Source: CAD feature listing. Evaluate the final solid. Frame: model axes, mm. A direction names the side the tool comes from. Give positions to 0.01 mm unless a question says otherwise; leave off trailing zeros. Loops run counter-clockwise (first coordinate to the right, second up) from the corner with the lowest first, then second, coordinate; pieces in that order, holes last. Notation, with made-up numbers: M -11,-40 L 5,-40 A27 ccw 5,-8 Z; hole C 53,82 d6. An arc over 180 degrees is marked long. Put each result on its own line as item: value.
from build123d import *

# Parameters (mm, degrees)
SKETCH1_W           = 28.2
SKETCH1_H           = 28.2
SKETCH1_R           = 11.1
SKETCH1_R_2         = 1.5
SKETCH1_R_3         = 5.2
BOSS_EXTRUDE1_DEPTH = 25
SKETCH1_4_R         = 5.2
CUT_EXTRUDE1_DEPTH  = 25
SKETCH1_5_R         = 1.5
CUT_EXTRUDE2_DEPTH  = 8
SKETCH1_6_R         = 11.1
SKETCH1_6_R_2       = 1.5
SKETCH1_6_R_3       = 5.2
CUT_EXTRUDE3_DEPTH  = 3.5
SKETCH2_R           = 1.5
CUT_EXTRUDE4_DEPTH  = 5


with BuildPart() as part:
    # Sketch1 → Boss-Extrude1 (new body)
    # profile 1 of 7: a face of its own
    with BuildSketch(Plane(origin=(0, 0, 0), x_dir=(1, 0, 0), z_dir=(0, 1, 0))):
        Rectangle(SKETCH1_W, SKETCH1_H)
        Circle(SKETCH1_R, mode=Mode.SUBTRACT)
    # profile 2 of 7: a face of its own
    with BuildSketch(Plane(origin=(0, 0, 0), x_dir=(1, 0, 0), z_dir=(0, 1, 0))):
        Circle(SKETCH1_R)
        with Locations((8, 0)):
            Circle(SKETCH1_R_2, mode=Mode.SUBTRACT)
        with Locations((0, -8)):
            Circle(SKETCH1_R_2, mode=Mode.SUBTRACT)
        with Locations((-8, 0)):
            Circle(SKETCH1_R_2, mode=Mode.SUBTRACT)
        with Locations((0, 8)):
            Circle(SKETCH1_R_2, mode=Mode.SUBTRACT)
        Circle(SKETCH1_R_3, mode=Mode.SUBTRACT)
    # profile 3 of 7: a face of its own
    with BuildSketch(Plane(origin=(0, 0, 0), x_dir=(1, 0, 0), z_dir=(0, 1, 0))):
        with Locations((0, 8)):
            Circle(SKETCH1_R_2)
    # profile 4 of 7: a face of its own
    with BuildSketch(Plane(origin=(0, 0, 0), x_dir=(1, 0, 0), z_dir=(0, 1, 0))):
        with Locations((8, 0)):
            Circle(SKETCH1_R_2)
    # profile 5 of 7: a face of its own
    with BuildSketch(Plane(origin=(0, 0, 0), x_dir=(1, 0, 0), z_dir=(0, 1, 0))):
        with Locations((0, -8)):
            Circle(SKETCH1_R_2)
    # profile 6 of 7: a face of its own
    with BuildSketch(Plane(origin=(0, 0, 0), x_dir=(1, 0, 0), z_dir=(0, 1, 0))):
        with Locations((-8, 0)):
            Circle(SKETCH1_R_2)
    # profile 7 of 7: a face of its own
    with BuildSketch(Plane(origin=(0, 0, 0), x_dir=(1, 0, 0), z_dir=(0, 1, 0))):
        Circle(SKETCH1_R_3)
    extrude(amount=BOSS_EXTRUDE1_DEPTH)

    # Sketch1_4 → Cut-Extrude1 (cut)
    with BuildSketch(Plane(origin=(0, 0, 0), x_dir=(1, 0, 0), z_dir=(0, 1, 0))):
        with Locations(Location((0, 0, 0), (0, 0, 270))):
            Circle(SKETCH1_4_R)
    extrude(amount=CUT_EXTRUDE1_DEPTH, mode=Mode.SUBTRACT)

    # Sketch1_5 → Cut-Extrude2 (cut)
    with BuildSketch(Plane(origin=(0, 0, 0), x_dir=(1, 0, 0), z_dir=(0, 1, 0))):
        with Locations(Location((-8, 0, 0), (0, 0, 270))):
            Circle(SKETCH1_5_R)
        with Locations(Location((0, -8, 0), (0, 0, 270))):
            Circle(SKETCH1_5_R)
        with Locations(Location((8, 0, 0), (0, 0, 270))):
            Circle(SKETCH1_5_R)
        with Locations(Location((0, 8, 0), (0, 0, 270))):
            Circle(SKETCH1_5_R)
    extrude(amount=CUT_EXTRUDE2_DEPTH, mode=Mode.SUBTRACT)

    # Sketch1_6 → Cut-Extrude3 (cut)
    with BuildSketch(Plane(origin=(0, 0, 0), x_dir=(1, 0, 0), z_dir=(0, 1, 0))):
        with Locations(Location((0, 0, 0), (0, 0, 270))):
            Circle(SKETCH1_6_R)
        with Locations(Location((8, 0, 0), (0, 0, 270))):
            Circle(SKETCH1_6_R_2, mode=Mode.SUBTRACT)
        with Locations(Location((0, -8, 0), (0, 0, 270))):
            Circle(SKETCH1_6_R_2, mode=Mode.SUBTRACT)
        with Locations(Location((-8, 0, 0), (0, 0, 270))):
            Circle(SKETCH1_6_R_2, mode=Mode.SUBTRACT)
        with Locations(Location((0, 8, 0), (0, 0, 270))):
            Circle(SKETCH1_6_R_2, mode=Mode.SUBTRACT)
        with Locations(Location((0, 0, 0), (0, 0, 270))):
            Circle(SKETCH1_6_R_3, mode=Mode.SUBTRACT)
    extrude(amount=CUT_EXTRUDE3_DEPTH, mode=Mode.SUBTRACT)

    # Sketch2 → Cut-Extrude4 (cut)
    with BuildSketch(Plane.ZY.offset(14.1)):
        with Locations((-7.5, 20.5)):
            Circle(SKETCH2_R)
        with Locations((7.5, 20.5)):
            Circle(SKETCH2_R)
        with Locations((7.5, 4.5)):
            Circle(SKETCH2_R)
        with Locations((-7.5, 4.5)):
            Circle(SKETCH2_R)
    extrude(amount=-CUT_EXTRUDE4_DEPTH, mode=Mode.SUBTRACT)


solid = part.part
1. Draft query along X for faces 1 (the cylindrical face through (-11.64, 21.51, -8.61)), 2 (the cylindrical face through (6.536, 5.719, -0.325)), 3 (the flat face through (-9.1, 21, 7)). Return one class per face: pulls with the +X half, pulls with the -X half, needs draft (parallel to the pull), parting line crosses it, or undercut.
Found:
face 1: needs draft
face 2: undercut
face 3: pulls with the -X half
2. Section query C-C (z = 0). Output: boundary loops of the cut face in (x, y).
Found:
outline: M -14.1,0 L -11.1,0 L -11.1,3.5 L -9.5,3.5 L -9.5,8 L -6.5,8 L -6.5,3.5 L -5.2,3.5 L -5.2,25 L -14.1,25 Z; M 5.2,3.5 L 6.5,3.5 L 6.5,8 L 9.5,8 L 9.5,3.5 L 11.1,3.5 L 11.1,0 L 14.1,0 L 14.1,25 L 5.2,25 Z
3. Material intervals for line 1 (X direction, y = 4.85, z = 0); line 2 (Y direction, x = -11.6, z = -7.5); line 3 (X direction, y = 0.7, z = 0), sorted ascending. Write a range as from..to.
Found:
line 1: -14.1..-9.5, -6.5..-5.2, 5.2..6.5, 9.5..14.1
line 2: 0..3, 6..19, 22..25
line 3: -14.1..-11.1, 11.1..14.1
4. Section query D-D (x = 8). Output: boundary loops of the cut face in (y, z).
Found:
outline: M 0,-14.1 L 25,-14.1 L 25,14.1 L 0,14.1 L 0,7.69 L 3.5,7.69 L 3.5,1.5 L 8,1.5 L 8,-1.5 L 3.5,-1.5 L 3.5,-7.69 L 0,-7.69 Z
5. Contact query for flat-ended pins moving along their axis: P1, Ø5, axis at x = 0, z = 8, coming from the -Y side; P2, Ø1.5, axis at y = 20.5, z = -7.5, coming from the -X side; P3, Ø6, axis at x = 0, z = 0, coming from the -Y side; P4, Ø1.5, axis at x = -7.5, z = 0, coming from the -Y side. Output: stop coordinate, or through.
Found:
P1: y = 3.5
P2: x = -9.1
P3: through
P4: y = 8
6. Section query A-A (y = 14.5). Output: boundary loops of the cut face in (x, z).
Found:
outline: M -14.1,-14.1 L 14.1,-14.1 L 14.1,14.1 L -14.1,14.1 Z; hole C 0,0 d10.4
7. Section query B-B (x = 4.5). Output: boundary loops of the cut face in (y, z).
Found:
outline: M 0,-14.1 L 25,-14.1 L 25,-2.61 L 3.5,-2.61 L 3.5,-10.15 L 0,-10.15 Z; M 0,10.15 L 3.5,10.15 L 3.5,2.61 L 25,2.61 L 25,14.1 L 0,14.1 Z
8. Access query for faces 4 (the flat face through (0, 8, -8)), 5 (the flat face through (14.1, 12, 0)), 6 (the cylindrical face through (-11.64, 21.51, 6.39)). Directions: +Z, -Z, +X, -X, +Y, -Y. A direction counts if a zero-diameter tool reaches every point of the face in a straight line with its end or side. Return the directions, or none.
Found:
face 4: -Y
face 5: +Z, -Z, +X, +Y, -Y
face 6: -X
